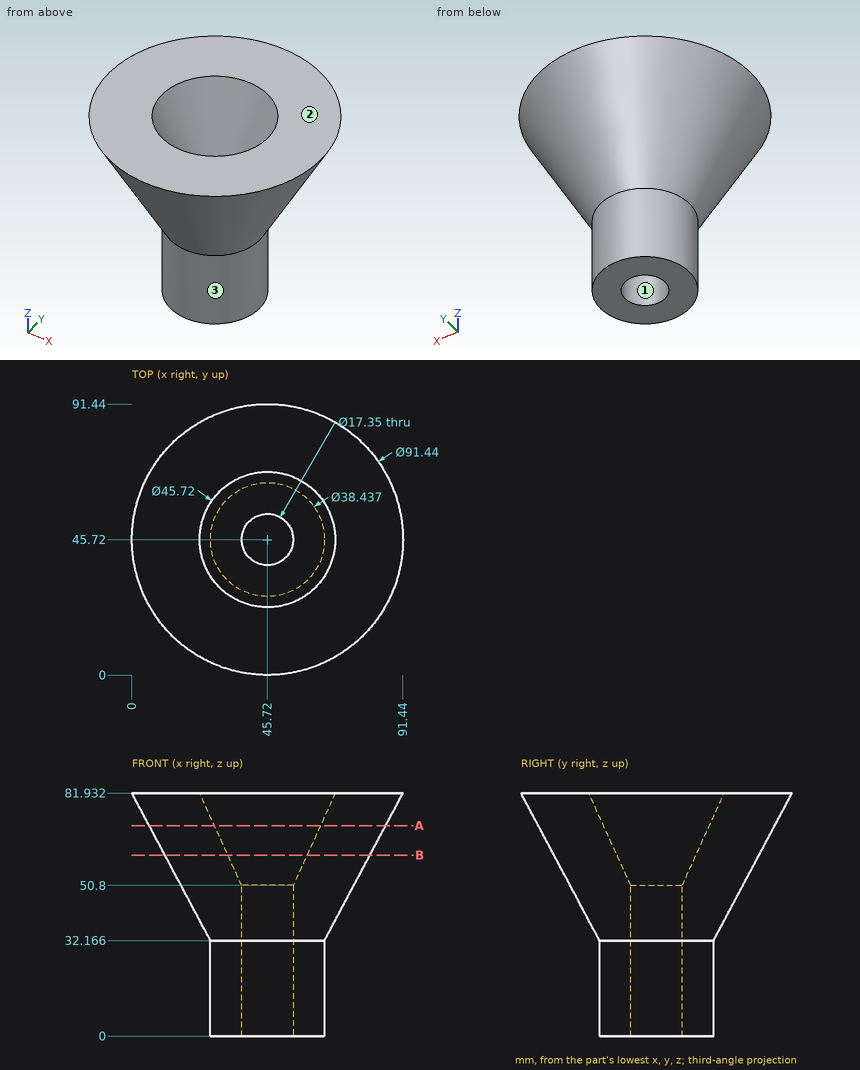
Verification items for this drawing (mm, ordinates from the low corner). Coordinates: 2 decimals unless noted, no trailing zeros. Order: outer loops, then holes, each group sorted by start corner. A loop starts at its lowest first (then second) coordinate and runs counter-clockwise, first axis right, second up.
Q1. Sectioned sample at B-B on z = 61. Record the cut outline in (x, y) (1 decimal).
Reply:
outline: circle Ø69.1 at (45.7, 45.7); hole circle Ø26.6 at (45.7, 45.7)
Q2. Sectioned sample at A-A on z = 71. Record the cut outline in (x, y), and give its area (3 significant figures).
Reply:
outline: circle Ø79.8 at (45.72, 45.72); hole circle Ø35.76 at (45.72, 45.72)
area: 4,000 mm2
Q3. Depth check by flat-ended pin: pin 1 Ø8 at (x, y) = (49, 21) entering from -Z; pin 2 Ø1 at (x, z) = (72, 68) entering from -Y; pin 3 Ø2 at (x, z) = (46, 38) entering from +Y. Enter the tip coordinate at first touch or a pass-through.
Reply:
pin 1: stops at z = 35.39
pin 2: stops at y = 17.27
pin 3: stops at y = 68.58
Q4. Thickness scan on probe 1 along X at (y, z) = (37.5, 61.5); probe 2 along Y at (x, z) = (51, 64.5); probe 3 along Y at (x, z) = (70, 50). Record the ranges inside material, lowest first.
Reply:
probe 1: x = 11.86 to 34.95, 56.49 to 79.58
probe 2: y = 9.67 to 31.77, 59.67 to 81.77
probe 3: y = 30.39 to 61.05
Q5. Draft check along Y on the marked faces 1, 2 and 3. Enter one of: released by +Y, released by -Y, zero draft, split by the parting line, or undercut.
Reply:
face 1: undercut
face 2: zero draft
face 3: split by the parting line
